```python
from build123d import *

# Parameters (mm, degrees)
SKETCH_R     = 2.5
SKETCH_R_2   = 5
SKETCH_R_3   = 1.5
PAD_DEPTH    = 5
CHAMFER_SIZE = 4


with BuildPart() as part:
    # Sketch → Pad (new body)
    with BuildSketch(Plane.XY):
        Polygon((84, 110.25), (44, 110.25), (0, 53.75), (0, 0), (84, 0), align=None)
        with Locations((15, 45.25)):
            Circle(SKETCH_R, mode=Mode.SUBTRACT)
        with Locations((15, 12.25)):
            Circle(SKETCH_R, mode=Mode.SUBTRACT)
        with Locations((15, 28.75)):
            Circle(SKETCH_R_2, mode=Mode.SUBTRACT)
        with Locations((53, 47)):
            Circle(SKETCH_R, mode=Mode.SUBTRACT)
        with Locations((53, 28.75)):
            Circle(SKETCH_R_2, mode=Mode.SUBTRACT)
        with Locations((53, 10.5)):
            Circle(SKETCH_R, mode=Mode.SUBTRACT)
        with Locations((54, 80.25)):
            Circle(SKETCH_R, mode=Mode.SUBTRACT)
        with Locations((74, 80.25)):
            Circle(SKETCH_R, mode=Mode.SUBTRACT)
        with Locations((54, 100.25)):
            Circle(SKETCH_R, mode=Mode.SUBTRACT)
        with Locations((74, 100.25)):
            Circle(SKETCH_R, mode=Mode.SUBTRACT)
        with Locations((74, 36.25)):
            Circle(SKETCH_R_3, mode=Mode.SUBTRACT)
        with Locations((74, 21.25)):
            Circle(SKETCH_R_3, mode=Mode.SUBTRACT)
    extrude(amount=PAD_DEPTH)

    # Chamfer
    chamfer_edges = [part.edges().sort_by_distance(p)[0] for p in [
        (0, 0, 2.5),
        (84, 0, 2.5),
    ]]
    chamfer(chamfer_edges, length=CHAMFER_SIZE)


solid = part.part
```
Here's how the part is built. I have some questions about the finished solid (model axes, mm). Coordinates: 2 decimals unless noted, no trailing zeros. Order: outer loops, then holes, each group sorted by start corner. A loop starts at its lowest first (then second) coordinate and runs counter-clockwise, first axis right, second up. Notation, with made-up numbers: M -30,-31 L 3,-31 A28 ccw 3,7 Z; hole C 13.25,-22.5 d7. An arc over 180 degrees is marked long. Answer as a JSON object with one key per item and string values. Group by question number.
(1) Suppose I cut it at A-A, the plane z = 2.6. State how many separate pieces and enclosed holes the cut face has, then the cut area to 3 significant figures.
(2) For pin 1 (10 mm diameter, centred on x = 61.5, y = 27.5, fed in from -Z); pin 2 (1.5 mm diameter, centred on y = 85, z = 0.5, fed in from -X), each with a flat end and sliding along its axis, tell me the tip position at first contact or that it passes through.
(3) Suppose I cut it at B-B, the plane x = 15. Please give me the cut outline in (y, z).
(4) Suppose I cut it at C-C, the plane y = 100.25. Please give me the cut outline in (x, z), then the cut area to 3 significant figures.
(5) I need wall thicknesses on probe 1 along Y at (x, z) = (74, 3.2); probe 2 along X at (y, z) = (81, 0.65); probe 3 along Y at (x, z) = (15, 2.9). Which ranges of each line are inside material? Lowest first, please.
(6) If we mould it in two halves opening along X, with no side actions, what happens to faces 1 (the face through (2, 2, 2)), 2 (the face through (75.386, 35.675, 2.465)), 3 (the face through (51, 56, 5))? For each: released by +X, released by -X, zero draft, split by the parting line, or undercut.
(7) Suppose I cut it at D-D, the plane x = 53. Please give me the cut outline in (y, z), then the cut area to 3 significant figures.
Values found:
{
 "1": {"separate pieces": "1", "enclosed holes": "12", "area": "7,670 mm^2"},
 "2": {"pin 1": "stops at z = 0", "pin 2": "stops at x = 23.75"},
 "3": {"outline": "M 0,0 L 9.75,0 L 9.75,5 L 0,5 Z; M 14.75,0 L 23.75,0 L 23.75,5 L 14.75,5 Z; M 33.75,0 L 42.75,0 L 42.75,5 L 33.75,5 Z; M 47.75,0 L 73.01,0 L 73.01,5 L 47.75,5 Z"},
 "4": {"outline": "M 36.21,0 L 51.5,0 L 51.5,5 L 36.21,5 Z; M 56.5,0 L 71.5,0 L 71.5,5 L 56.5,5 Z; M 76.5,0 L 84,0 L 84,5 L 76.5,5 Z", "area": "189 mm^2"},
 "5": {"probe 1": "y = 0 to 19.75, 22.75 to 34.75, 37.75 to 77.75, 82.75 to 97.75, 102.75 to 110.25", "probe 2": "x = 21.22 to 51.62, 56.38 to 71.62, 76.38 to 84", "probe 3": "y = 0 to 9.75, 14.75 to 23.75, 33.75 to 42.75, 47.75 to 73.01"},
 "6": {"face 1": "released by -X", "face 2": "undercut", "face 3": "zero draft"},
 "7": {"outline": "M 0,0 L 8,0 L 8,5 L 0,5 Z; M 13,0 L 23.75,0 L 23.75,5 L 13,5 Z; M 33.75,0 L 44.5,0 L 44.5,5 L 33.75,5 Z; M 49.5,0 L 77.96,0 L 77.96,5 L 49.5,5 Z; M 82.54,0 L 97.96,0 L 97.96,5 L 82.54,5 Z; M 102.54,0 L 110.25,0 L 110.25,5 L 102.54,5 Z", "area": "405 mm^2"}
}
